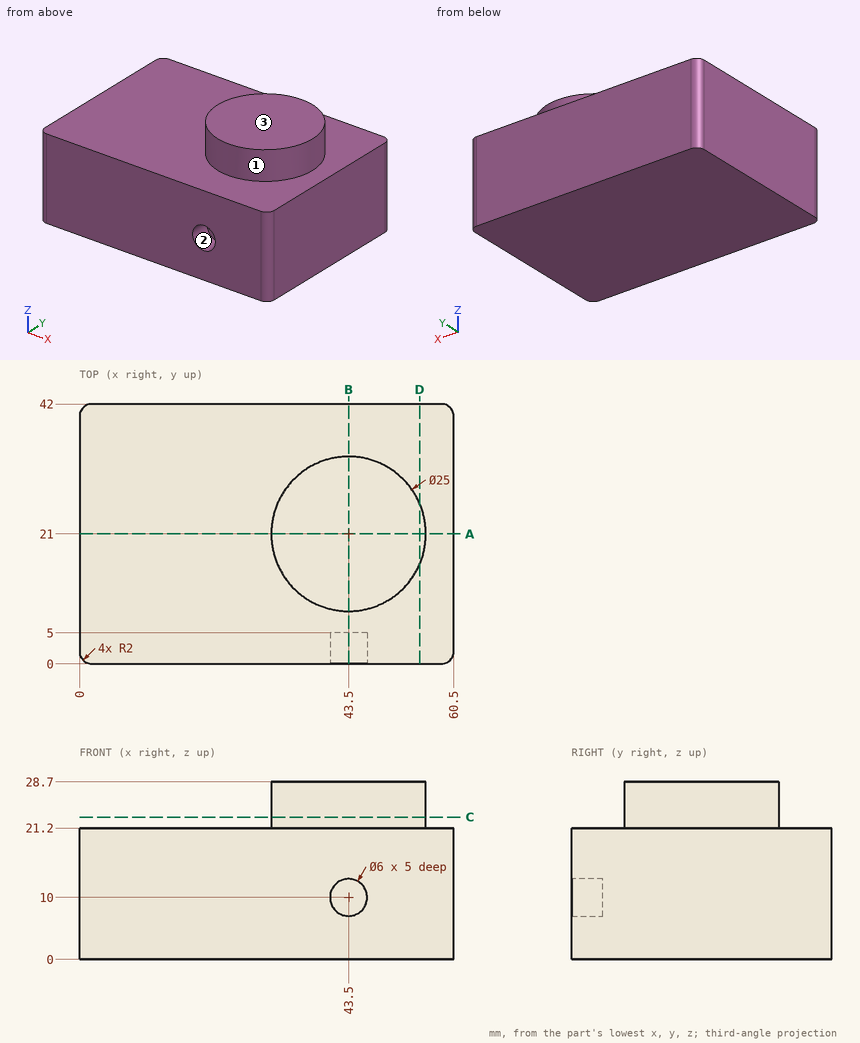
Input: dimensioned drawing with shaded views. Units: mm. Origin: part minimum x, y, z. Round coordinates to 2 decimals unless told otherwise and drop trailing zeros. Order: outer loops, then holes, each group sorted by start corner. A loop starts at its lowest first (then second) coordinate and runs counter-clockwise, first axis right, second up. Notation, with made-up numbers: M -20.5,-8.5 L 4.5,-8.5 A16 ccw 4.5,0.5 Z; hole C -30.5,-10 d9. An arc over 180 degrees is marked long. Use one line per item in the form item = value. Start each with the question number.
Q1. Material intervals for line 1 (X direction, y = 1.9, z = 10); line 2 (Z direction, x = 43, y = 1); line 3 (Z direction, x = 24.5, y = 34.5), sorted ascending. Write a range as [from, to].
Q2. Cut plane C-C (z = 23). Return loops of the section in (x, y).
Q3. Cut plane D-D (x = 55). Return loops of the section in (y, z), and give its area (3 significant figures).
Q4. Pin query (flat end, axial travel): pin 1 Ø6.5 at (x, z) = (43.5, 8.5) entering from -Y; pin 2 Ø10 at (x, y) = (9.5, 31) entering from +Z. Return the tip coordinate at first contact, or that it passes through.
Q5. Cut plane B-B (x = 43.5). Return loops of the section in (y, z).
Q6. Cut plane A-A (y = 21). Return loops of the section in (x, z), and give its area (3 significant figures).
Q7. Mould query, pull axis Z, two halves, no side actions, for the marked faces 1, 2 and 3. Classes: +Z half, -Z half, draft (parallel to the pull), parting line (faces both ways), or undercut.
Geometry results:
q1.line_1 = [0, 40.5], [46.5, 60.5]
q1.line_2 = [0, 7.04], [12.96, 21.2]
q1.line_3 = [0, 21.2]
q2.outline = C 43.5,21 d25
q3.outline = M 0,0 L 42,0 L 42,21.2 L 25.9,21.2 L 25.9,28.7 L 16.1,28.7 L 16.1,21.2 L 0,21.2 Z
q3.area = 964 mm^2
q4.pin_1 = 0
q4.pin_2 = 21.2
q5.outline = M 0,0 L 42,0 L 42,21.2 L 33.5,21.2 L 33.5,28.7 L 8.5,28.7 L 8.5,21.2 L 0,21.2 L 0,13 L 5,13 L 5,7 L 0,7 Z
q6.outline = M 0,0 L 60.5,0 L 60.5,21.2 L 56,21.2 L 56,28.7 L 31,28.7 L 31,21.2 L 0,21.2 Z
q6.area = 1,470 mm^2
q7.face_1 = draft
q7.face_2 = undercut
q7.face_3 = +Z half
